```python
from build123d import *

# Parameters (mm, degrees)
SKETCH1_W           = 150
SKETCH1_H           = 60
SKETCH1_W_2         = 2.5
SKETCH1_H_2         = 10
SKETCH1_W_3         = 20
SKETCH1_H_3         = 2.5
BOSS_EXTRUDE1_DEPTH = 2.5
FILLET2_R           = 2


with BuildPart() as part:
    # Sketch1 → Boss-Extrude1 (new body)
    with BuildSketch(Plane.XY):
        Rectangle(SKETCH1_W, SKETCH1_H)
        with Locations((-71.75, -15)):
            Rectangle(SKETCH1_W_2, SKETCH1_H_2, mode=Mode.SUBTRACT)
        with Locations((-71.75, 15)):
            Rectangle(SKETCH1_W_2, SKETCH1_H_2, mode=Mode.SUBTRACT)
        with Locations((0, 15)):
            Rectangle(SKETCH1_W_2, SKETCH1_H_2, mode=Mode.SUBTRACT)
        with Locations((0, -15)):
            Rectangle(SKETCH1_W_2, SKETCH1_H_2, mode=Mode.SUBTRACT)
        with Locations((71.75, 15)):
            Rectangle(SKETCH1_W_2, SKETCH1_H_2, mode=Mode.SUBTRACT)
        with Locations((71.75, -15)):
            Rectangle(SKETCH1_W_2, SKETCH1_H_2, mode=Mode.SUBTRACT)
        with Locations((0, -26.75)):
            Rectangle(SKETCH1_W_3, SKETCH1_H_3, mode=Mode.SUBTRACT)
        with Locations((-55, -26.75)):
            Rectangle(SKETCH1_W_3, SKETCH1_H_3, mode=Mode.SUBTRACT)
        with Locations((55, -26.75)):
            Rectangle(SKETCH1_W_3, SKETCH1_H_3, mode=Mode.SUBTRACT)
    extrude(amount=BOSS_EXTRUDE1_DEPTH)

    # Fillet2
    fillet2_edges = [part.edges().sort_by_distance(p)[0] for p in [
        (75, -30, 1.25),
        (-75, -30, 1.25),
        (-75, 30, 1.25),
        (75, 30, 1.25),
    ]]
    fillet(fillet2_edges, radius=FILLET2_R)


solid = part.part
```
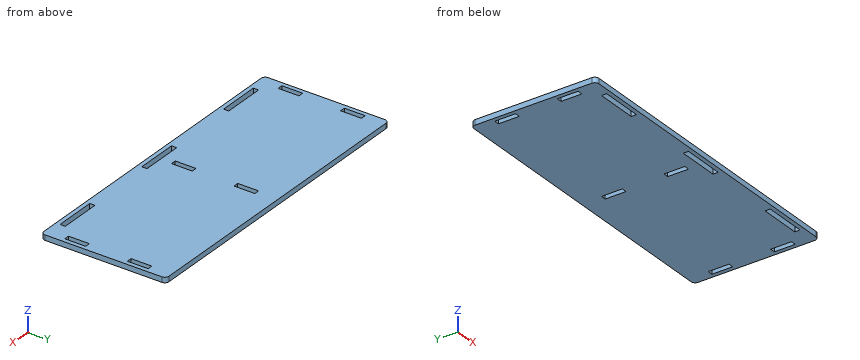
Work out the finished part from the listing and answer in its coordinate system (mm). Give positions to 0.01 mm unless a question says otherwise; leave off trailing zeros. Order: outer loops, then holes, each group sorted by start corner. A loop starts at its lowest first (then second) coordinate and runs counter-clockwise, first axis right, second up. Notation, with made-up numbers: M -14.5,-32 L 10.5,-32 A17 ccw 10.5,-16 Z; hole C -18.5,16 d10. An arc over 180 degrees is marked long. Return JSON: item names as keys, results as strings.
1) Section C-C, the plane z = 1.3 is taken. Give the number of separate pieces and of enclosed holes in the cut face, plus the area to 3 significant figures.
Resolved:
{"separate pieces": "1", "enclosed holes": "9", "area": "8,700 mm^2"}
2) Straight lines are drawn through the part: line 1 along X through (y, z) = (10.5, 1.75); line 2 along Y through (x, z) = (-52, 0.95). For each, find the intervals that lie inside material, in ascending order. Write a range as [from, to].
Resolved:
{"line 1": "[-75, -73], [-70.5, -1.25], [1.25, 70.5], [73, 75]", "line 2": "[-30, -28], [-25.5, 30]"}
3) Section A-A, the plane y = -18 is taken. Write down the section's boundary in (x, z), plus the area to 3 significant figures.
Resolved:
{"outline": "M -75,0 L -73,0 L -73,2.5 L -75,2.5 Z; M -70.5,0 L -1.25,0 L -1.25,2.5 L -70.5,2.5 Z; M 1.25,0 L 70.5,0 L 70.5,2.5 L 1.25,2.5 Z; M 73,0 L 75,0 L 75,2.5 L 73,2.5 Z", "area": "356 mm^2"}
4) Section B-B, the plane x = 57 is taken. Write down the section's boundary in (y, z), plus the area to 3 significant figures.
Resolved:
{"outline": "M -30,0 L -28,0 L -28,2.5 L -30,2.5 Z; M -25.5,0 L 30,0 L 30,2.5 L -25.5,2.5 Z", "area": "144 mm^2"}
